Build history of the part. All positions in model axes, mm. Face numbers are marked on the shaded views. A direction names the side the tool comes from. Give positions to 0.01 mm unless a question says otherwise; leave off trailing zeros. Order: outer loops, then holes, each group sorted by start corner. A loop starts at its lowest first (then second) coordinate and runs counter-clockwise, first axis right, second up. Notation, with made-up numbers: (88.25, 35.25) - (123.25, 35.25) arc R14 ccw to (123.25, 51.25) - close; hole circle Ø2 at (1, -31). An arc over 180 degrees is marked (long way). Use a Markdown table: item, result. Add a question column.
(1) Slice it at D-D (y = -7.75). Write the cut outline in (x, z).
(2) Slice it at C-C (y = -1.75). Write the cut outline in (x, z), then the cut area to 3 significant figures.
(3) Flat gauge pins, fed straight in: pin 1 (6.5 mm diameter, centred on y = -8.5, z = 34.5, fed in from +X); pin 2 (8 mm diameter, centred on y = -8.5, z = 11, fed in from +X); pin 3 (8 mm diameter, centred on x = 7, z = 26, fed in from +Y); pin 4 (2 mm diameter, centred on x = 16, y = -14, fed in from -Z). Where does each tip first touch, or does it go through?
(4) Slice it at A-A (x = 0). Write the cut outline in (y, z).
(5) Which spindle directions (+Z, -Z, +X, -X, +Y, -Y) get a long thin tool onto all of the face, cutting with end or side? Do the marked faces 1, 2, 3, 4 and 5. Say none if no direction does.
(6) Wall check: line 1 (X direction, y = -12.5, z = 4.5); line 2 (Z direction, x = -25, y = -6). Give the ranges that are in metal, low to high.
(7) Slice it at B-B (z = 6). Write the cut outline in (x, y).
from build123d import *

# Parameters (mm, degrees)
F1_DEPTH = 2.54
F3_DEPTH = 19.05
F4_SIZE  = 1.27
F5_R     = 7.62


with BuildPart() as f1:
    # F0 (on Front) → F1 (new body)
    with BuildSketch(Plane.XZ):
        with BuildLine():
            Line((-31.75, 38.1), (-31.75, 0))
            Line((-31.75, 0), (31.75, 0))
            Line((31.75, 0), (31.75, 38.1))
            Line((31.75, 38.1), (12.7, 38.1))
            ThreePointArc((12.7, 38.1), (0, 25.4), (-12.7, 38.1))
            Line((-12.7, 38.1), (-31.75, 38.1))
        make_face()
    extrude(amount=F1_DEPTH)

    # F2 (on face) → F3 (join)
    with BuildSketch(Plane.XZ.offset(2.54)):
        with BuildLine():
            Line((19.05, 0), (25.4, 0))
            Line((25.4, 0), (25.4, 15.761378))
            ThreePointArc((25.4, 15.761378), (18.249038, 18.397703), (15.24, 25.4))
            Line((15.24, 25.4), (15.24, 38.1))
            Line((15.24, 38.1), (12.7, 38.1))
            ThreePointArc((12.7, 38.1), (0, 25.4), (-12.7, 38.1))
            Line((-12.7, 38.1), (-15.24, 38.1))
            Line((-15.24, 38.1), (-15.24, 25.4))
            ThreePointArc((-15.24, 25.4), (-18.249038, 18.397703), (-25.4, 15.761378))
            Line((-25.4, 15.761378), (-25.4, 0))
            Line((-25.4, 0), (-19.05, 0))
            Line((-19.05, 0), (-19.05, 10.16))
            Line((-19.05, 10.16), (19.05, 10.16))
            Line((19.05, 10.16), (19.05, 0))
        make_face()
    extrude(amount=F3_DEPTH)

    # F4
    f4_edges = [f1.edges().sort_by_distance(p)[0] for p in [
        (0, -21.59, 10.16),
        (-19.05, -21.59, 5.08),
        (19.05, -21.59, 5.08),
        (0, -21.59, 25.4),
    ]]
    chamfer(f4_edges, length=F4_SIZE)

    # F5
    f5_edges = [f1.edges().sort_by_distance(p)[0] for p in [
        (-31.75, -1.27, 38.1),
        (31.75, -1.27, 38.1),
    ]]
    fillet(f5_edges, radius=F5_R)


solid = f1.part
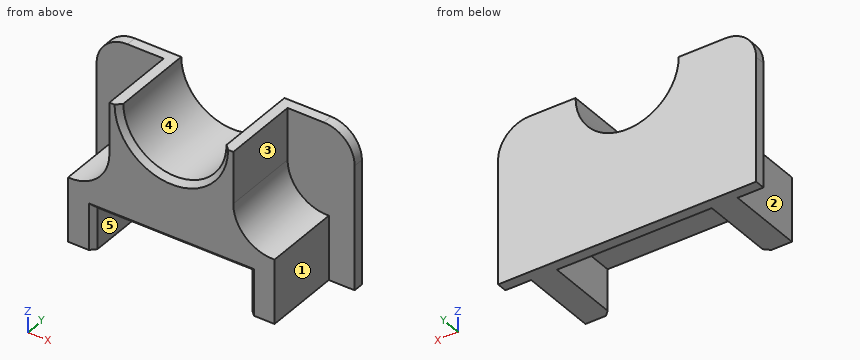
Solution:
| question | item | result |
|---|---|---|
| 1 | outline | (-25.4, 0) - (-19.05, 0) - (-19.05, 10.16) - (19.05, 10.16) - (19.05, 0) - (25.4, 0) - (25.4, 15.76) arc R9.65 cw to (15.24, 25.4) - (15.24, 38.1) - (12.7, 38.1) arc R12.7 cw to (-12.7, 38.1) - (-15.24, 38.1) - (-15.24, 25.4) arc R9.65 cw to (-25.4, 15.76) - close |
| 2 | outline | (-31.75, 0) - (31.75, 0) - (31.75, 30.48) arc R7.62 ccw to (24.13, 38.1) - (12.7, 38.1) arc R12.7 cw to (-12.7, 38.1) - (-24.13, 38.1) arc R7.62 ccw to (-31.75, 30.48) - close |
| 2 | area | 2,140 mm2 |
| 3 | pin 1 | x = 15.24 |
| 3 | pin 2 | x = 25.4 |
| 3 | pin 3 | y = 0 |
| 3 | pin 4 | z = 10.16 |
| 4 | outline | (-21.59, 11.43) - (-20.32, 10.16) - (-2.54, 10.16) - (-2.54, 0) - (0, 0) - (0, 25.4) - (-20.32, 25.4) - (-21.59, 24.13) - close |
| 5 | face 1 | +Z, -Z, +X, -Y |
| 5 | face 2 | +Z, -Z, -X, -Y |
| 5 | face 3 | +Z, +X, -Y |
| 5 | face 4 | +Z, +Y, -Y |
| 5 | face 5 | -Z, -Y |
| 6 | line 1 | -25.4 to -19.05, 19.05 to 25.4 |
| 6 | line 2 | 0 to 15.75 |
| 7 | outline | (-31.75, -2.54) - (-25.4, -2.54) - (-25.4, -21.59) - (-20.32, -21.59) - (-19.05, -20.32) - (-19.05, -2.54) - (19.05, -2.54) - (19.05, -20.32) - (20.32, -21.59) - (25.4, -21.59) - (25.4, -2.54) - (31.75, -2.54) - (31.75, 0) - (-31.75, 0) - close |
